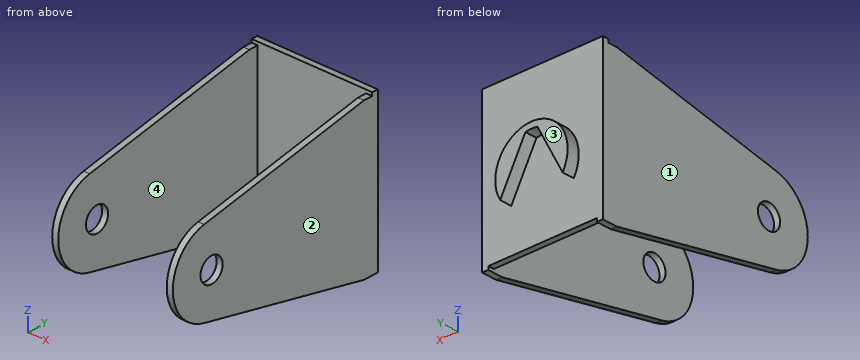
```python
from build123d import *

# Parameters (mm, degrees)
BOSS_EXTRUDE1_DEPTH = 2
SKETCH2_W           = 40
SKETCH2_H           = 50
BOSS_EXTRUDE2_DEPTH = 2
BOSS_EXTRUDE3_DEPTH = 4
SKETCH4_R           = 4
CUT_EXTRUDE1_DEPTH  = 41


with BuildPart() as part:
    # Sketch1 → Boss-Extrude1 (new body)
    with BuildSketch(Plane(origin=(0, 0, 0), x_dir=(0, 0, -1), z_dir=(1, 0, 0))):
        with BuildLine():
            Line((-4.485924614, 52.27530577), (6.773398514, -5.406820081))
            ThreePointArc((6.773398514, -5.406820081), (20.514075386, -16.72469423), (34.254752259, -5.406820081))
            Line((34.254752259, -5.406820081), (45.514075386, 52.27530577))
            Line((45.514075386, 52.27530577), (45.514075386, 57.27530577))
            Line((45.514075386, 57.27530577), (-4.485924614, 57.27530577))
            Line((-4.485924614, 57.27530577), (-4.485924614, 52.27530577))
        make_face()
    extrude(amount=-BOSS_EXTRUDE1_DEPTH)


with BuildPart() as body_2:
    # Mirror1: mirrored copy
    add(part.part.mirror(Plane(origin=(-20, 0, 0), x_dir=(0, 0, 1), z_dir=(1, 0, 0))))


with BuildPart() as part_1:
    add(part.part)

    add(body_2.part)  # Boss-Extrude2 merges body 2
    # Sketch2 → Boss-Extrude2 (add)
    with BuildSketch(Plane(origin=(0, 57.27530577, 0), x_dir=(1, 0, 0), z_dir=(0, 1, 0))):
        with Locations((-20, 19.454333817)):
            Rectangle(SKETCH2_W, SKETCH2_H)
    extrude(amount=-BOSS_EXTRUDE2_DEPTH)

    # Sketch3 → Boss-Extrude3 (add)
    with BuildSketch(Plane(origin=(0, 57.27530577, 0), x_dir=(1, 0, 0), z_dir=(0, 1, 0))):
        with BuildLine():
            Line((-18, 14.653938589), (-9.643842411, 30.514075386))
            ThreePointArc((-9.643842411, 30.514075386), (-20, 12.45189756), (-30.356157589, 30.514075386))
            Line((-30.356157589, 30.514075386), (-22, 14.653938589))
            ThreePointArc((-22, 14.653938589), (-20, 14.45189756), (-18, 14.653938589))
        make_face()
    extrude(amount=BOSS_EXTRUDE3_DEPTH)

    # Sketch4 → Cut-Extrude1 (cut, through all)
    with BuildSketch(Plane(origin=(0, 0, 0), x_dir=(0, 0, -1), z_dir=(1, 0, 0))):
        with Locations((20.514075386, -2.72469423)):
            Circle(SKETCH4_R)
    extrude(amount=-CUT_EXTRUDE1_DEPTH, mode=Mode.SUBTRACT)


solid = part_1.part
```
Model file for the job. Use its own axes, mm. Face numbers are marked on the shaded views. Coordinates: 2 decimals unless noted, no trailing zeros. Order: outer loops, then holes, each group sorted by start corner. A loop starts at its lowest first (then second) coordinate and runs counter-clockwise, first axis right, second up. Notation, with made-up numbers: (68.25, 39.25) -> (126.25, 39.25) arc R19 cw to (126.25, 76.25) -> close; hole circle Ø10 at (58.25, 47). An arc over 180 degrees is marked (long way). Return JSON: item names as keys, results as strings.
Item 1: Mould opens along X. For the marked faces 1, 2, 3 and 4 say: pulls with the +X half, pulls with the -X half, needs draft (parallel to the pull), parting line crosses it, or undercut.
Model answer:
{"face 1": "pulls with the -X half", "face 2": "pulls with the +X half", "face 3": "needs draft", "face 4": "undercut"}
Item 2: Slice it at B-B (x = -20). Write the cut outline in (y, z), then the cut area to 3 significant figures.
Model answer:
{"outline": "(55.28, -44.45) -> (57.28, -44.45) -> (57.28, -14.45) -> (61.28, -14.45) -> (61.28, -12.45) -> (57.28, -12.45) -> (57.28, 5.55) -> (55.28, 5.55) -> close", "area": "108 mm²"}
Item 3: Slice it at D-D (y = 14). Write the cut outline in (x, z).
Model answer:
{"outline": "(-40, -38.04) -> (-38, -38.04) -> (-38, -2.99) -> (-40, -2.99) -> close; (-2, -38.04) -> (0, -38.04) -> (0, -2.99) -> (-2, -2.99) -> close"}
Item 4: Pin check, flat tips, straight feed: P1, Ø1.6, axis at x = -17.5, y = 56, coming from the -Z side; P2, Ø4, axis at x = -9, z = -40.5, coming from the +Y side; P3, Ø12, axis at x = -26, z = -32.5, coming from the -Y side. Stop position of each tip, or through.
Model answer:
{"P1": "stops at z = -44.45", "P2": "stops at y = 57.28", "P3": "stops at y = 55.28"}
Item 5: Slice it at C-C (z = -10). Write the cut outline in (x, y).
Model answer:
{"outline": "(-40, -11.97) -> (-38, -11.97) -> (-38, 55.28) -> (-2, 55.28) -> (-2, -11.97) -> (0, -11.97) -> (0, 57.28) -> (-40, 57.28) -> close"}
Item 6: Wall check: line 1 along X through (y, z) = (50, -11.5); line 2 along Z through (x, y) = (-9, 57); line 3 along Y through (x, z) = (-14, 0). Give the ranges that are in metal, low to high. Write a range as from..to.
Model answer:
{"line 1": "x = -40..-38, -2..0", "line 2": "z = -44.45..5.55", "line 3": "y = 55.28..57.28"}
Item 7: Slice it at A-A (y = -10). Write the cut outline in (x, z), then the cut area to 3 significant figures.
Model answer:
{"outline": "(-40, -32.48) -> (-38, -32.48) -> (-38, -8.55) -> (-40, -8.55) -> close; (-2, -32.48) -> (0, -32.48) -> (0, -8.55) -> (-2, -8.55) -> close", "area": "95.7 mm²"}
